Check sheet for the modelled part. Datum: model origin and axes. Units: mm. A direction names the side the tool comes from. Round coordinates to 2 decimals unless told otherwise and drop trailing zeros. Write each loop counter-clockwise with the first axis right and the second up, starting at its lowest first coordinate (ties: lowest second). Pieces come first, ordered by that corner, then holes. Notation, with made-up numbers: M -31,15.25 L 11,15.25 A21 ccw 11,54.25 Z; hole C -40,-37 d11. An arc over 180 degrees is marked long. Answer in a Markdown table with one row per item.
```python
from build123d import *

# Parameters (mm, degrees)
SKETCH1_R           = 0.75
BOSS_EXTRUDE1_DEPTH = 10


with BuildPart() as part:
    # Sketch1 → Boss-Extrude1 (new body)
    with BuildSketch(Plane.XY):
        with BuildLine():
            Line((12.147549978, 2.281559418), (6.5, 1))
            Line((6.5, 1), (0.852450022, 2.281559418))
            ThreePointArc((0.852450022, 2.281559418), (-1.975, 0.5), (0.852450022, -1.281559418))
            Line((0.852450022, -1.281559418), (6.5, 0))
            Line((6.5, 0), (12.147549978, -1.281559418))
            ThreePointArc((12.147549978, -1.281559418), (14.975, 0.5), (12.147549978, 2.281559418))
        make_face()
        with Locations((0, 0.5)):
            Circle(SKETCH1_R, mode=Mode.SUBTRACT)
        with Locations((13, 0.5)):
            Circle(SKETCH1_R, mode=Mode.SUBTRACT)
    extrude(amount=BOSS_EXTRUDE1_DEPTH)


solid = part.part
```
1. Scan lines: L1, parallel to X at y = 0.45, z = 6; L2, parallel to X at y = 0.15, z = 6.5; L3, parallel to Y at x = 13, z = 5 (3 decimals). Record each from-to range of solid material in increasing order.
Found:
| item | result |
|---|---|
| L1 | x = -1.97 to -0.75, 0.75 to 12.25, 13.75 to 14.97 |
| L2 | x = -1.94 to -0.66, 0.66 to 12.34, 13.66 to 14.94 |
| L3 | y = -1.475 to -0.25, 1.25 to 2.475 |
2. Section check D-D, the plane x = 8.5. Record the cut outline in (y, z).
Found:
| item | result |
|---|---|
| outline | M -0.45,0 L 1.45,0 L 1.45,10 L -0.45,10 Z |
3. Section check C-C, the plane y = 0.5. Record the cut outline in (x, z) (3 decimals).
Found:
| item | result |
|---|---|
| outline | M -1.975,0 L -0.75,0 L -0.75,10 L -1.975,10 Z; M 0.75,0 L 12.25,0 L 12.25,10 L 0.75,10 Z; M 13.75,0 L 14.975,0 L 14.975,10 L 13.75,10 Z |
4. Draft check along X on faces 1 (the face through (6.4, 0.5, 10)), 2 (the face through (-1.974, 0.556, 4.93)). Enter one of: +X half, -X half, draft (parallel to the pull), parting line (faces both ways), or undercut.
Found:
| item | result |
|---|---|
| face 1 | draft |
| face 2 | undercut |
5. Go/stop test with flat-tipped pins: pin 1 (2 mm diameter, centred on x = 1.5, z = 1.5, fed in from -Y); pin 2 (2 mm diameter, centred on y = 2, z = 7.5, fed in from -X); pin 3 (6 mm diameter, centred on x = 4.5, z = 5, fed in from -Y); pin 4 (1.4 mm diameter, centred on x = 0, y = 0.5, fed in from +Z). Record where each tip stops, or that it passes through.
Found:
| item | result |
|---|---|
| pin 1 | stops at y = -1.41 |
| pin 2 | stops at x = -1.91 |
| pin 3 | stops at y = -1.13 |
| pin 4 | passes through |
6. Access from +Z, -Z, +X, -X, +Y, -Y to the whole of each face (thin tool, end or side, straight path). Record for faces 3 (the face through (3.72, 1.63, 4.93)), 4 (the face through (6.4, 0.5, 0)), 5 (the face through (3.64, -0.65, 4.93)).
Found:
| item | result |
|---|---|
| face 3 | +Z, -Z, +Y |
| face 4 | -Z, +X, -X, +Y, -Y |
| face 5 | +Z, -Z, -Y |
7. Section check B-B, the plane z = 7.5. Record the cut outline in (x, y) (3 decimals).
Found:
| item | result |
|---|---|
| outline | M 0.852,-1.282 L 6.5,0 L 12.148,-1.282 A1.975 ccw long 12.148,2.282 L 6.5,1 L 0.852,2.282 A1.975 ccw long Z; hole C 0,0.5 d1.5; hole C 13,0.5 d1.5 |
8. Section check A-A, the plane x = 0. Record the cut outline in (y, z) (3 decimals).
Found:
| item | result |
|---|---|
| outline | M -1.475,0 L -0.25,0 L -0.25,10 L -1.475,10 Z; M 1.25,0 L 2.475,0 L 2.475,10 L 1.25,10 Z |
